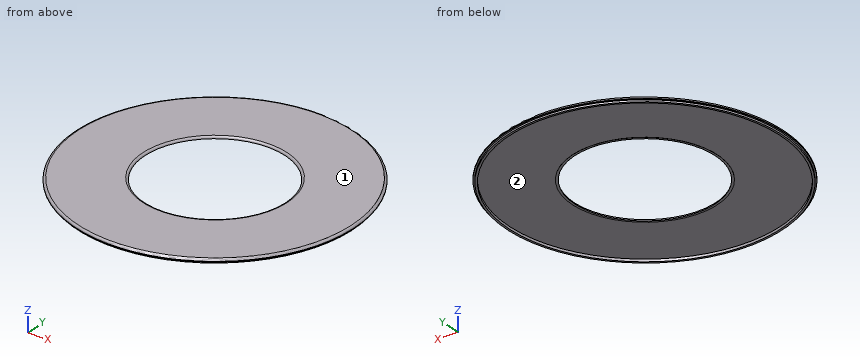
```python
from build123d import *


# Not quite as in the source:
# - a fillet or chamfer that OpenCascade refuses, or shapes differently, is made with other operations: its cross-section is extruded or revolved along the edge and cut away or added


with BuildPart() as f1:
    # F0 (on Front) → F1 (revolve)
    with BuildSketch(Plane.XZ):
        Polygon((118, 0), (59.5, 0), (59.5, -1.75), (61.45, -1.75), (61.45, -1.65), (114.95, -1.65), (114.95, -3.75), (116.7, -3.75), (116.7, -2.25), (118, -2.25), align=None)
    revolve(axis=Axis((0, 0, -2.4080555886), (0, 0, -1)))

    # F2: fillet of radius 1.8 on 2 edges, made by hand

    # F2_s1 → F2_t2 (revolve, cut)
    with BuildSketch(Plane.XZ):
        with BuildLine():
            ThreePointArc((61.3, 0), (60.0272077939, -0.5272077939), (59.5, -1.8))
            Line((59.5, -1.8), (59.5, 0))
            Line((59.5, 0), (61.3, 0))
        make_face()
    revolve(axis=Axis((0, 0, 0), (0, 0, -1)), mode=Mode.SUBTRACT)

    # F2_s3 → F2_t4 (revolve, cut)
    with BuildSketch(Plane.XZ):
        with BuildLine():
            ThreePointArc((116.2, 0), (117.4727922061, -0.5272077939), (118, -1.8))
            Line((118, -1.8), (118, 0))
            Line((118, 0), (116.2, 0))
        make_face()
    revolve(axis=Axis((0, 0, 0), (0, 0, -1)), mode=Mode.SUBTRACT)


solid = f1.part
```
Check sheet for the modelled part. Datum: model origin and axes. Units: mm. Face numbers are marked on the shaded views. Coordinates: 2 decimals unless noted, no trailing zeros. Write each loop counter-clockwise with the first axis right and the second up, starting at its lowest first coordinate (ties: lowest second). Pieces come first, ordered by that corner, then holes. Notation, with made-up numbers: (1, 23) - (12, 23) arc R6 cw to (12, 31) - close; hole circle Ø10 at (-39.5, -26.75). An arc over 180 degrees is marked (long way). One line per question, with ' | ' between items.
Item 1: Gauge pin test, flat end, axial feed: P1, Ø1, axis at y = 73, z = -2.5, coming from the -X side. Record the tip position at first contact, or that the pin passes through.
Determined:
P1: stops at x = -93.05
Item 2: Mould release check, pull along Y, two halves, no side actions. Record for the marked faces 1 and 2: pulls with the +Y half, pulls with the -Y half, needs draft (parallel to the pull), parting line crosses it, or undercut.
Determined:
face 1: needs draft | face 2: undercut
Item 3: Sectioned sample at A-A on y = 0. Record the boundary of the cut face in (x, z).
Determined:
outline: (-118, -2.25) - (-116.7, -2.25) - (-116.7, -3.75) - (-114.95, -3.75) - (-114.95, -1.65) - (-61.45, -1.65) - (-61.45, -1.75) - (-59.5, -1.75) arc R1.8 ccw to (-61.3, 0) - (-116.2, 0) arc R1.8 ccw to (-118, -1.8) - close; (59.5, -1.75) - (61.45, -1.75) - (61.45, -1.65) - (114.95, -1.65) - (114.95, -3.75) - (116.7, -3.75) - (116.7, -2.25) - (118, -2.25) - (118, -1.8) arc R1.8 ccw to (116.2, 0) - (61.3, 0) arc R1.8 ccw to start
Item 4: Thickness scan on line 1 (X direction, y = 0, z = -2.4); line 2 (X direction, y = -41.5, z = -1.7). Record the ranges inside material, lowest first. Write a range as [from, to].
Determined:
line 1: x = [-116.7, -114.95], [114.95, 116.7] | line 2: x = [-110.46, -107.2], [-45.32, -42.64], [42.64, 45.32], [107.2, 110.46]
Item 5: Sectioned sample at C-C on z = -0.85. Record the boundary of the cut face in (x, y).
Determined:
outline: circle Ø235.46 at (0, 0); hole circle Ø119.54 at (0, 0)
